Design review of the part built by this model. Coordinates are the model's own, in mm. Face numbers are marked on the shaded views. A direction names the side the tool comes from. Coordinates: 2 decimals unless noted, no trailing zeros. Order: outer loops, then holes, each group sorted by start corner. A loop starts at its lowest first (then second) coordinate and runs counter-clockwise, first axis right, second up. Notation, with made-up numbers: (86, -29) -> (112, -29) arc R25 ccw to (112, 2) -> close; hole circle Ø4 at (42.5, -2.75). An arc over 180 degrees is marked (long way). Write item = value, one per line.
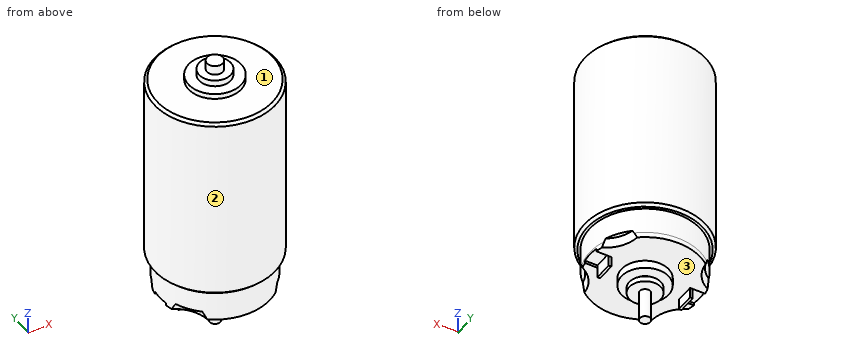
```python
from build123d import *

# Parameters (mm, degrees)
CROQUIS1_R                      = 11.5
SALIENTE_EXTRUIR1_DEPTH         = 36
CROQUIS1_4_R                    = 5
SALIENTE_EXTRUIR2_DEPTH         = 1
CROQUIS1_5_R                    = 3
SALIENTE_EXTRUIR3_DEPTH         = 2.2
CROQUIS1_6_R                    = 1.5
SALIENTE_EXTRUIR4_DEPTH         = 4
CROQUIS3_R                      = 10.5
SALIENTE_EXTRUIR5_DEPTH         = 5
CROQUIS7_R                      = 10.5
SALIENTE_EXTRUIR10_DEPTH        = 1
CROQUIS3_6_R                    = 1
SALIENTE_EXTRUIR7_DEPTH         = 14.8
SALIENTE_EXTRUIR8_START         = 9.1
CROQUIS3_8_R                    = 3
SALIENTE_EXTRUIR8_DEPTH         = 9.1
CROQUIS3_9_R                    = 4.5
SALIENTE_EXTRUIR9_DEPTH         = 7.5
CROQUIS5_W                      = 0.55
CROQUIS5_H                      = 0.6
CORTAR_EXTRUIR1_DEPTH           = 1.5
CORTAR_EXTRUIR1_DRAFT           = -20
CORTAR_EXTRUIR1_PROFILE_2_DEPTH = 1.5
CORTAR_EXTRUIR1_PROFILE_2_DRAFT = -20
CORTAR_EXTRUIR1_PROFILE_3_DEPTH = 1.5
CORTAR_EXTRUIR1_PROFILE_3_DRAFT = -20
CORTAR_EXTRUIR1_PROFILE_4_DEPTH = 1.5
CORTAR_EXTRUIR1_PROFILE_4_DRAFT = -20
CHAFL_N1_SIZE                   = 0.5
CORTAR_EXTRUIR2_START           = -0.5
CORTAR_EXTRUIR2_DEPTH           = 0.5
CROQUIS10_W                     = 0.5
CROQUIS10_H                     = 3.5
SALIENTE_EXTRUIR11_DEPTH        = 2.5


with BuildPart() as part:
    # Croquis1 → Saliente-Extruir1 (new body)
    with BuildSketch(Plane.XY):
        Circle(CROQUIS1_R)
    extrude(amount=-SALIENTE_EXTRUIR1_DEPTH)

    # Croquis1<4> → Saliente-Extruir2 (add)
    with BuildSketch(Plane.XY):
        Circle(CROQUIS1_4_R)
    extrude(amount=SALIENTE_EXTRUIR2_DEPTH)

    # Croquis1<5> → Saliente-Extruir3 (add)
    with BuildSketch(Plane.XY):
        Circle(CROQUIS1_5_R)
    extrude(amount=SALIENTE_EXTRUIR3_DEPTH)

    # Croquis1<6> → Saliente-Extruir4 (add)
    with BuildSketch(Plane.XY):
        Circle(CROQUIS1_6_R)
    extrude(amount=SALIENTE_EXTRUIR4_DEPTH)

    # Croquis3 → Saliente-Extruir5 (add)
    with BuildSketch(Plane(origin=(0, 0, -36), x_dir=(-1, 0, 0), z_dir=(0, 0, -1))):
        Circle(CROQUIS3_R)
    extrude(amount=SALIENTE_EXTRUIR5_DEPTH)

    # Croquis3<6> → Saliente-Extruir7 (add)
    with BuildSketch(Plane(origin=(0, 0, -36), x_dir=(-1, 0, 0), z_dir=(0, 0, -1))):
        Circle(CROQUIS3_6_R)
    extrude(amount=SALIENTE_EXTRUIR7_DEPTH)

    # Croquis3<8> → Saliente-Extruir8 (add)
    with BuildSketch(Plane(origin=(0, 0, -36), x_dir=(-1, 0, 0), z_dir=(0, 0, -1)).offset(SALIENTE_EXTRUIR8_START)):
        with Locations(Location((0, 0, 0), (0, 0, 180))):
            Circle(CROQUIS3_8_R)
    extrude(amount=-SALIENTE_EXTRUIR8_DEPTH)

    # Croquis3<9> → Saliente-Extruir9 (add)
    with BuildSketch(Plane(origin=(0, 0, -36), x_dir=(-1, 0, 0), z_dir=(0, 0, -1))):
        Circle(CROQUIS3_9_R)
    extrude(amount=SALIENTE_EXTRUIR9_DEPTH)

    # Cortar-Barrer1: sweep along a curve in space
    with BuildLine() as cortar_barrer1_path:
        ThreePointArc((-3, 0, -45.1), (-2.121320344, 2.121320344, -45.1), (0, 3, -45.1))
        ThreePointArc((0, 3, -45.1), (2.121320344, 2.121320344, -45.1), (3, 0, -45.1))
        ThreePointArc((3, 0, -45.1), (2.121320344, -2.121320344, -45.1), (0, -3, -45.1))
        ThreePointArc((0, -3, -45.1), (-2.121320344, -2.121320344, -45.1), (-3, 0, -45.1))
    # Croquis5 → Cortar-Barrer1 (sweep, cut)
    with BuildSketch(Plane(origin=(0, 0, 0), x_dir=(0, 0, -1), z_dir=(1, 0, 0))):
        with Locations((43.775, 2.7)):
            Rectangle(CROQUIS5_W, CROQUIS5_H)
    sweep(path=cortar_barrer1_path.line, mode=Mode.SUBTRACT)


with BuildPart() as body_2:
    # Croquis7 → Saliente-Extruir10 (new body)
    with BuildSketch(Plane(origin=(0, 0, -41), x_dir=(-1, 0, 0), z_dir=(0, 0, -1))):
        Circle(CROQUIS7_R)
    extrude(amount=SALIENTE_EXTRUIR10_DEPTH)


with BuildPart() as cortar_extruir1_tool:
    # Croquis8 → Cortar-Extruir1 (with draft: the straight prism first)
    with BuildSketch(Plane(origin=(0, 0, -42), x_dir=(-1, 0, 0), z_dir=(0, 0, -1))):
        with BuildLine():
            ThreePointArc((-6.51000025, -9.479973457), (-7.597986649, -5.15921898), (-11.212760015, -2.554214724))
            ThreePointArc((-11.212760015, -2.554214724), (-9.513968223, -6.460217384), (-6.51000025, -9.479973457))
        make_face()
    extrude(amount=-CORTAR_EXTRUIR1_DEPTH)
    # Cortar-Extruir1: the draft: its side faces are tilted about the plane it starts from
    cortar_extruir1_sides = [cortar_extruir1_tool.faces().sort_by_distance(p)[0] for p in [
        (7.597986649, -5.15921898, -41.25),
        (9.513968223, -6.460217384, -41.25),
    ]]
    draft(cortar_extruir1_sides, Plane(origin=(0, 0, -42), x_dir=(-1, 0, 0), z_dir=(0, 0, -1)), CORTAR_EXTRUIR1_DRAFT)


with BuildPart() as part_1:
    add(part.part)

    # Cortar-Extruir1: cut by cortar_extruir1_tool
    add(cortar_extruir1_tool.part, mode=Mode.SUBTRACT)


with BuildPart() as body_2_1:
    add(body_2.part)

    # Cortar-Extruir1: cut by cortar_extruir1_tool
    add(cortar_extruir1_tool.part, mode=Mode.SUBTRACT)


with BuildPart() as cortar_extruir1_profile_2_tool:
    # Croquis8 → Cortar-Extruir1 profile 2 (with draft: the straight prism first)
    with BuildSketch(Plane(origin=(0, 0, -42), x_dir=(-1, 0, 0), z_dir=(0, 0, -1))):
        with BuildLine():
            ThreePointArc((-6.51000025, 9.479973457), (-9.513968223, 6.460217384), (-11.212760015, 2.554214724))
            ThreePointArc((-11.212760015, 2.554214724), (-7.597986649, 5.15921898), (-6.51000025, 9.479973457))
        make_face()
    extrude(amount=-CORTAR_EXTRUIR1_PROFILE_2_DEPTH)
    # Cortar-Extruir1 profile 2: the draft: its side faces are tilted about the plane it starts from
    cortar_extruir1_profile_2_sides = [cortar_extruir1_profile_2_tool.faces().sort_by_distance(p)[0] for p in [
        (9.513968223, 6.460217384, -41.25),
        (7.597986649, 5.15921898, -41.25),
    ]]
    draft(cortar_extruir1_profile_2_sides, Plane(origin=(0, 0, -42), x_dir=(-1, 0, 0), z_dir=(0, 0, -1)), CORTAR_EXTRUIR1_PROFILE_2_DRAFT)


with BuildPart() as part_2:
    add(part_1.part)

    # Cortar-Extruir1 profile 2: cut by cortar_extruir1_profile_2_tool
    add(cortar_extruir1_profile_2_tool.part, mode=Mode.SUBTRACT)


with BuildPart() as body_2_2:
    add(body_2_1.part)

    # Cortar-Extruir1 profile 2: cut by cortar_extruir1_profile_2_tool
    add(cortar_extruir1_profile_2_tool.part, mode=Mode.SUBTRACT)


with BuildPart() as cortar_extruir1_profile_3_tool:
    # Croquis8 → Cortar-Extruir1 profile 3 (with draft: the straight prism first)
    with BuildSketch(Plane(origin=(0, 0, -42), x_dir=(-1, 0, 0), z_dir=(0, 0, -1))):
        with BuildLine():
            ThreePointArc((6.51000025, 9.479973457), (7.597986649, 5.15921898), (11.212760015, 2.554214724))
            ThreePointArc((11.212760015, 2.554214724), (9.513968223, 6.460217384), (6.51000025, 9.479973457))
        make_face()
    extrude(amount=-CORTAR_EXTRUIR1_PROFILE_3_DEPTH)
    # Cortar-Extruir1 profile 3: the draft: its side faces are tilted about the plane it starts from
    cortar_extruir1_profile_3_sides = [cortar_extruir1_profile_3_tool.faces().sort_by_distance(p)[0] for p in [
        (-9.513968223, 6.460217384, -41.25),
        (-7.597986649, 5.15921898, -41.25),
    ]]
    draft(cortar_extruir1_profile_3_sides, Plane(origin=(0, 0, -42), x_dir=(-1, 0, 0), z_dir=(0, 0, -1)), CORTAR_EXTRUIR1_PROFILE_3_DRAFT)


with BuildPart() as part_3:
    add(part_2.part)

    # Cortar-Extruir1 profile 3: cut by cortar_extruir1_profile_3_tool
    add(cortar_extruir1_profile_3_tool.part, mode=Mode.SUBTRACT)


with BuildPart() as body_2_3:
    add(body_2_2.part)

    # Cortar-Extruir1 profile 3: cut by cortar_extruir1_profile_3_tool
    add(cortar_extruir1_profile_3_tool.part, mode=Mode.SUBTRACT)


with BuildPart() as cortar_extruir1_profile_4_tool:
    # Croquis8 → Cortar-Extruir1 profile 4 (with draft: the straight prism first)
    with BuildSketch(Plane(origin=(0, 0, -42), x_dir=(-1, 0, 0), z_dir=(0, 0, -1))):
        with BuildLine():
            ThreePointArc((6.51000025, -9.479973457), (9.513968223, -6.460217384), (11.212760015, -2.554214724))
            ThreePointArc((11.212760015, -2.554214724), (7.597986649, -5.15921898), (6.51000025, -9.479973457))
        make_face()
    extrude(amount=-CORTAR_EXTRUIR1_PROFILE_4_DEPTH)
    # Cortar-Extruir1 profile 4: the draft: its side faces are tilted about the plane it starts from
    cortar_extruir1_profile_4_sides = [cortar_extruir1_profile_4_tool.faces().sort_by_distance(p)[0] for p in [
        (-7.597986649, -5.15921898, -41.25),
        (-9.513968223, -6.460217384, -41.25),
    ]]
    draft(cortar_extruir1_profile_4_sides, Plane(origin=(0, 0, -42), x_dir=(-1, 0, 0), z_dir=(0, 0, -1)), CORTAR_EXTRUIR1_PROFILE_4_DRAFT)


with BuildPart() as part_4:
    add(part_3.part)

    # Cortar-Extruir1 profile 4: cut by cortar_extruir1_profile_4_tool
    add(cortar_extruir1_profile_4_tool.part, mode=Mode.SUBTRACT)

    # Chaflán1
    chafl_n1_edges = [part_4.edges().sort_by_distance(p)[0] for p in [
        (-11.5, 0, 0),
        (-11.5, 0, -36),
    ]]
    chamfer(chafl_n1_edges, length=CHAFL_N1_SIZE)



with BuildPart() as body_2_4:
    add(body_2_3.part)

    # Cortar-Extruir1 profile 4: cut by cortar_extruir1_profile_4_tool
    add(cortar_extruir1_profile_4_tool.part, mode=Mode.SUBTRACT)

    # Croquis9 → Cortar-Extruir2 (cut)
    with BuildSketch(Plane(origin=(0, 0, -42), x_dir=(-1, 0, 0), z_dir=(0, 0, -1)).offset(CORTAR_EXTRUIR2_START)):
        with BuildLine():
            Line((-10.35313962, -1.75), (-8, -1.75))
            Line((-8, -1.75), (-7.5, -1.75))
            Line((-7.5, -1.75), (-7.5, 1.75))
            Line((-7.5, 1.75), (-8, 1.75))
            Line((-8, 1.75), (-10.35313962, 1.75))
            ThreePointArc((-10.35313962, 1.75), (-10.463220489, 0.878075733), (-10.5, 0))
            ThreePointArc((-10.5, 0), (-10.463220489, -0.878075733), (-10.35313962, -1.75))
        make_face()
        with BuildLine():
            Line((7.5, -1.75), (8, -1.75))
            Line((8, -1.75), (10.35313962, -1.75))
            ThreePointArc((10.35313962, -1.75), (10.463220489, -0.878075733), (10.5, 0))
            ThreePointArc((10.5, 0), (10.463220489, 0.878075733), (10.35313962, 1.75))
            Line((10.35313962, 1.75), (8, 1.75))
            Line((8, 1.75), (7.5, 1.75))
            Line((7.5, 1.75), (7.5, -1.75))
        make_face()
    extrude(amount=CORTAR_EXTRUIR2_DEPTH, mode=Mode.SUBTRACT)


with BuildPart() as part_5:
    add(part_4.part)

    add(body_2_4.part)  # Saliente-Extruir11 merges body 2
    # Croquis10 → Saliente-Extruir11 (add)
    with BuildSketch(Plane(origin=(0, 0, -41.5), x_dir=(-1, 0, 0), z_dir=(0, 0, -1))):
        with Locations((7.75, 0)):
            Rectangle(CROQUIS10_W, CROQUIS10_H)
        with Locations((-7.75, 0)):
            Rectangle(CROQUIS10_W, CROQUIS10_H)
    extrude(amount=SALIENTE_EXTRUIR11_DEPTH)


solid = part_5.part
```
(1) We need section A-A (z = -14). Write out the cut boundary in (x, y), and give its area (3 significant figures).
Report:
outline = circle Ø23 at (0, 0)
area = 415 mm²
(2) For L1, parallel to Y at x = 1.75, z = -41.5; L2, parallel to Z at x = -2, y = -2.5; L3, parallel to Z at x = -5.5, y = -1.25, list the stretches that pass through material, from the lowest coordinate up.
Report:
L1 = -10.35 to 10.35
L2 = -43.5 to 1
L3 = -42 to 0
(3) Insertion check: pin 1 (0.6 mm diameter, centred on x = -8, y = 0.5, fed in from -Z); pin 2 (6 mm diameter, centred on y = -8.5, z = -29, fed in from -X); pin 3 (3 mm diameter, centred on x = -10, y = 0.5, fed in from -Z). Each pin has a flat end and moves straight along its axis. Give the tip position at first contact, or say it passes through.
Report:
pin_1 = -44
pin_2 = -10.1
pin_3 = -42
(4) For the marked faces 1, 2 and 3, list the 3-axis set-ups (+Z, -Z, +X, -X, +Y, -Y) from which the entire face can be reached by the end or side of a thin tool; tool diameter is ignored.
Report:
face_1 = +Z
face_2 = +Z, -Z
face_3 = -Z
